from build123d import *

# Parameters (mm, degrees)
EXTRUDE_1_DEPTH     = 6.5
CUT_EXTRUDE_1_DEPTH = 52.886896226
CUT_EXTRUDE_2_DEPTH = 54.09425581


with BuildPart() as part:
    # 草图1 → 凸台-拉伸1 (new, symmetric)
    with BuildSketch(Plane(origin=(0, 0, 0), x_dir=(1, 0, 0), z_dir=(0, 1, 0))):
        with BuildLine():
            Line((0, 0), (0, 6))
            ThreePointArc((0, 6), (7.402826909, 27.529174564), (22, 45))
            Line((22, 45), (25, 45))
            Line((25, 45), (25, 42))
            ThreePointArc((25, 42), (21.416586692, 24), (25, 6))
            Line((25, 6), (20, 6))
            Line((20, 6), (20, 0))
            Line((20, 0), (0, 0))
        make_face()
    extrude(amount=EXTRUDE_1_DEPTH, both=True)

    # 草图3 → 切除-拉伸1 (cut, through all)
    with BuildSketch(Plane.ZY):
        Polygon((0, 4), (0, 6.5), (-4.253461365, 6.5), (-4.253461365, 3.25), align=None)
        Polygon((0, -4), (-4.253461365, -3.25), (-4.253461365, -6.5), (0, -6.5), align=None)
    extrude(amount=-CUT_EXTRUDE_1_DEPTH, mode=Mode.SUBTRACT)

    # 草图4 → 切除-拉伸2 (cut, through all)
    with BuildSketch(Plane(origin=(0, 6.5, 0), x_dir=(1, 0, 0), z_dir=(0, 1, 0))):
        with BuildLine():
            ThreePointArc((7.169736852, 12.07909507), (12.400276965, 12.65373917), (17.63523501, 12.120841452))
            ThreePointArc((17.63523501, 12.120841452), (19.45114939, 12.654920589), (20.008524733, 14.463820333))
            ThreePointArc((20.008524733, 14.463820333), (19.071107342, 24.389014044), (20.121422197, 34.302896243))
            ThreePointArc((20.121422197, 34.302896243), (19.130864623, 36.4613018), (16.77629627, 36.151581393))
            ThreePointArc((16.77629627, 36.151581393), (9.141463638, 26.201122888), (4.785137328, 14.439970103))
            ThreePointArc((4.785137328, 14.439970103), (5.336190032, 12.611841621), (7.169736852, 12.07909507))
        make_face()
    extrude(amount=-CUT_EXTRUDE_2_DEPTH, mode=Mode.SUBTRACT)


solid = part.part
Input: part model. Units: mm. Frame: model coordinates. A direction names the side the tool comes from. Round coordinates to 2 decimals unless told otherwise and drop trailing zeros. Loops run counter-clockwise (first coordinate to the right, second up) from the corner with the lowest first, then second, coordinate; pieces in that order, holes last. Notation, with made-up numbers: (-15.5, -16.75) -> (-5.5, -16.75) arc R15 ccw to (-5.5, 6.25) -> close; hole circle Ø2 at (43, 13). An arc over 180 degrees is marked (long way). Answer as a JSON object with one key per item and string values. Group by question number.
1) Pin query (flat end, axial travel): pin 1 (5 mm diameter, centred on y = -3, z = -4, fed in from +X); pin 2 (1.5 mm diameter, centred on y = -4.5, z = -38.5, fed in from +X); pin 3 (1 mm diameter, centred on x = 11, y = 5.5, fed in from +Z). Return the tip coordinate at first contact, or that it passes through.
2) Reachability of faces 1 (the flat face through (10, 5, -4.253)), 2 (the flat face through (23, 0, -6)), 3 (the cylindrical face through (12.326, 0.091, -12.653)), 4 (the flat face through (10, -5, -4.253)) from +Z, -Z, +X, -X, +Y, -Y: full face, straight path, thin tool, end or side. Return the list, or none.
3) Section query D-D on x = 13.75. Output: boundary loops of the cut face in (y, z), plus the area to 3 significant figures.
4) Section query C-C on y = 1.75. Output: boundary loops of the cut face in (x, z), plus the area to 3 significant figures.
5) Section query B-B on z = -17. Output: boundary loops of the cut face in (x, y).
6) Ray query, L1, parallel to X at y = 3, z = -15; L2, parallel to X at y = -3, z = -36; L3, parallel to Z at x = 18.75, y = 0.5. Return the intervals inside material, ascending.
7) Section query A-A on x = 11. Output: boundary loops of the cut face in (y, z), plus the area to 3 significant figures.
8) Draft query along Z for faces 5 (the flat face through (20, 0, -4)), 6 (the cylindrical face through (9.23, 0.09, -26.36)), 7 (the flat face through (23, 0, -45)). Return one class per face: +Z half, -Z half, draft (parallel to the pull), parting line (faces both ways), or undercut.
Reply:
{
 "1": {"pin 1": "stops at x = 25", "pin 2": "stops at x = 23.96", "pin 3": "stops at z = -4.25"},
 "2": {"face 1": "+X, -X, +Y", "face 2": "+Z, +X, +Y, -Y", "face 3": "+Y, -Y", "face 4": "+X, -X, -Y"},
 "3": {"outline": "(-6.5, -36.75) -> (6.5, -36.75) -> (6.5, -32.91) -> (-6.5, -32.91) -> close; (-6.5, -12.62) -> (6.5, -12.62) -> (6.5, -4.25) -> (3.25, -4.25) -> (4, 0) -> (-4, 0) -> (-3.25, -4.25) -> (-6.5, -4.25) -> close", "area": "190 mm2"},
 "4": {"outline": "(0, -6) arc R62.75 ccw to (22, -45) -> (25, -45) -> (25, -42) arc R47 cw to (25, -6) -> (20, -6) -> (20, 0) -> (0, 0) -> close; hole (4.79, -14.44) arc R42 ccw to (16.78, -36.15) arc R2 ccw to (20.12, -34.3) arc R50 cw to (20.01, -14.46) arc R2 ccw to (17.64, -12.12) arc R25 cw to (7.17, -12.08) arc R2 ccw to start", "area": "453 mm2"},
 "5": {"outline": "(2.68, -6.5) -> (5.4, -6.5) -> (5.4, 6.5) -> (2.68, 6.5) -> close; (19.58, -6.5) -> (21.94, -6.5) -> (21.94, 6.5) -> (19.58, 6.5) -> close"},
 "6": {"L1": "x = 2.03 to 4.91, 19.91 to 22.29", "L2": "x = 13.14 to 16.62, 19.69 to 22.97", "L3": "z = -42.11 to -36.62, -12.21 to 0"},
 "7": {"outline": "(-6.5, -33.18) -> (6.5, -33.18) -> (6.5, -29.25) -> (-6.5, -29.25) -> close; (-6.5, -12.61) -> (6.5, -12.61) -> (6.5, -4.25) -> (3.25, -4.25) -> (4, 0) -> (-4, 0) -> (-3.25, -4.25) -> (-6.5, -4.25) -> close", "area": "191 mm2"},
 "8": {"face 5": "draft", "face 6": "undercut", "face 7": "-Z half"}
}
